The model under review builds one solid part; all positions refer to its coordinate system, in mm. Face numbers are marked on the shaded views. A direction names the side the tool comes from. Round coordinates to 2 decimals unless told otherwise and drop trailing zeros. Loops run counter-clockwise (first coordinate to the right, second up) from the corner with the lowest first, then second, coordinate; pieces in that order, holes last. Notation, with made-up numbers: (-22.5, -31.75) -> (-13.5, -31.75) arc R19 ccw to (-13.5, -17.75) -> close; hole circle Ø7 at (27, 28.5). An arc over 180 degrees is marked (long way). Return JSON: item names as keys, results as strings. Group by question number.
```python
from build123d import *

# Parameters (mm, degrees)
F0_W     = 152.4
F0_H     = 63.5
F1_DEPTH = 31.75
F3_W     = 152.4
F3_H     = 15.875
F4_DEPTH = 19.05
F2_W     = 152.4
F2_H     = 15.875
F5_DEPTH = 19.05
F7_R     = 14.2875
F8_DEPTH = 31.751


with BuildPart() as f1:
    # F0 (on Top) → F1 (new body)
    with BuildSketch(Plane.XY):
        with Locations((1.061699, -22.131501)):
            Rectangle(F0_W, F0_H)
    extrude(amount=F1_DEPTH)

    # F3 (on face) → F4 (join)
    with BuildSketch(Plane.XZ.offset(53.881501)):
        with Locations((1.061699, 23.8125)):
            Rectangle(F3_W, F3_H)
    extrude(amount=F4_DEPTH)

    # F2 (on face) → F5 (join)
    with BuildSketch(Plane(origin=(0, 9.618499, 0), x_dir=(-1, 0, 0), z_dir=(0, 1, 0))):
        with Locations((-1.061699, 23.8125)):
            Rectangle(F2_W, F2_H)
    extrude(amount=F5_DEPTH)

    # F7 (on face) → F8 (cut, through all)
    with BuildSketch(Plane(origin=(0, 0, 0), x_dir=(1, 0, 0), z_dir=(0, 0, -1))):
        with Locations((1.310549, 19.654326)):
            Circle(F7_R)
    extrude(amount=-F8_DEPTH, mode=Mode.SUBTRACT)


solid = f1.part
```
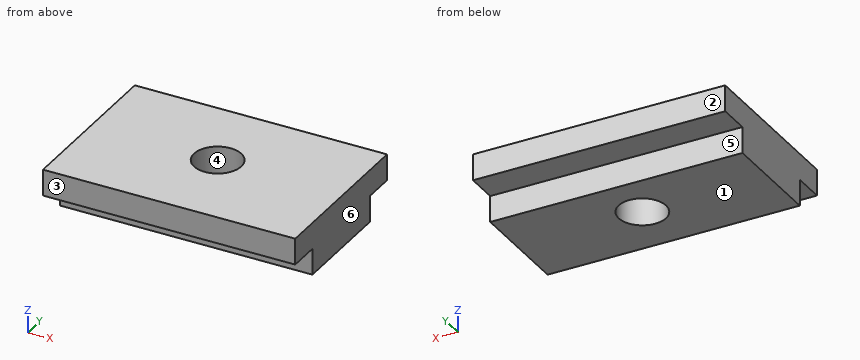
1. Wall thickness on line 1 (X direction, y = -31, z = 22); line 2 (X direction, y = -10, z = 10); line 3 (Y direction, x = -50, z = 8.5): over which ranges is each line inside the solid? List them lowest first.
2. Tool access review of the marked faces 5 and 6: name each direction out of +Z, -Z, +X, -X, +Y, -Y from which nothing blocks a thin tool from reaching the whole face with its end or side.
3. We need section B-B, the plane y = -29.5. Write out the cut boundary in (x, z), then the cut area to 3 significant figures.
4. We need section D-D, the plane z = 18.5. Write out the cut boundary in (x, y) (1 decimal), then the cut area to 3 significant figures.
5. Draft analysis for pull direction Y (two halves, no side actions). For the marked faces 1, 2, 3 and 4, state which applies: pulls with the +Y half, pulls with the -Y half, needs draft (parallel to the pull), parting line crosses it, or undercut.
6. For P1, Ø8, axis at x = -6.5, z = 8, coming from the +Y side; P2, Ø2, axis at x = 20, z = 3.5, coming from the -Y side; P3, Ø9.5, axis at x = 9.5, y = 21.5, coming from the -Z side (3 decimals); P4, Ø17, axis at x = 1.31, y = -19.65, coming from the +Z side, all flat-tipped, find the tip position at first contact; note any pin that passes through.
7. We need section C-C, the plane y = -64.5. Write out the cut boundary in (x, z) (3 decimals), then the cut area to 3 significant figures.
Check sheet entries:
{
 "1": {"line 1": "x = -75.14 to -7.37, 9.99 to 77.26", "line 2": "x = -75.14 to -9.22, 11.84 to 77.26", "line 3": "y = -53.88 to 9.62"},
 "2": {"face 5": "-Z, +X, -X, +Y", "face 6": "+Z, -Z, +X, +Y, -Y"},
 "3": {"outline": "(-75.14, 0) -> (-9.04, 0) -> (-9.04, 31.75) -> (-75.14, 31.75) -> close; (11.66, 0) -> (77.26, 0) -> (77.26, 31.75) -> (11.66, 31.75) -> close", "area": "4,180 mm²"},
 "4": {"outline": "(-75.1, -72.9) -> (77.3, -72.9) -> (77.3, 28.7) -> (-75.1, 28.7) -> close; hole circle Ø28.6 at (1.3, -19.7)", "area": "14,800 mm²"},
 "5": {"face 1": "needs draft", "face 2": "pulls with the +Y half", "face 3": "pulls with the -Y half", "face 4": "undercut"},
 "6": {"P1": "stops at y = 9.62", "P2": "stops at y = -53.88", "P3": "stops at z = 15.875", "P4": "passes through"},
 "7": {"outline": "(-75.138, 15.875) -> (77.262, 15.875) -> (77.262, 31.75) -> (-75.138, 31.75) -> close", "area": "2,420 mm²"}
}
